from build123d import *

# Parameters (mm, degrees)
PAD066_DEPTH            = 57.4
POCKET083_DEPTH         = 4.5
SKETCH144_R             = 3.1
POCKET097_DEPTH         = 10
POCKET097_FACE16_W      = 10
POCKET097_FACE16_H      = 57.4
PAD073_DEPTH            = 6.35
SKETCH147_R             = 1.85
POCKET099_DEPTH         = 57.401
BODY017_PLACEMENT_ANGLE = 270


with BuildPart() as part:
    # Sketch126 → Pad066 (new body)
    with BuildSketch(Plane.XY):
        with BuildLine():
            Line((10, 10), (10, 60))
            Line((10, 60), (0, 60))
            Line((0, 60), (0, 0))
            add(Edge.make_bspline(
                [(0, 0), (45, -90), (90, 0)],
                knots=[0, 0, 0, 1, 1, 1], degree=2))
            Line((90, 0), (90, 60))
            Line((90, 60), (80, 60))
            Line((80, 60), (80, 10))
            add(Edge.make_bspline(
                [(10, 10), (45, -60), (80, 10)],
                knots=[0, 0, 0, 1, 1, 1], degree=2))
        make_face()
    extrude(amount=PAD066_DEPTH)

    # Sketch127 (on Face1 of Pad066) → Pocket083 (cut)
    with BuildSketch(Plane.YZ.offset(10)):
        Polygon((28.425, 33.679646), (25.55, 28.7), (28.425, 23.720354), (34.175, 23.720354), (37.05, 28.7), (34.175, 33.679646), align=None)
    extrude(amount=-POCKET083_DEPTH, mode=Mode.SUBTRACT)

    # Sketch144 (on Face13 of Pocket083) → Pocket097 (cut)
    with BuildSketch(Plane(origin=(0, 0, 0), x_dir=(0, -1, 0), z_dir=(-1, 0, 0))):
        with Locations((-31.3, 28.7)):
            Circle(SKETCH144_R)
    extrude(amount=-POCKET097_DEPTH, mode=Mode.SUBTRACT)

    # Pocket097 Face16 → Pad073 (add)
    with BuildSketch(Plane(origin=(85, 60, 28.7), x_dir=(1, 0, 0), z_dir=(0, 1, 0))):
        Rectangle(POCKET097_FACE16_W, POCKET097_FACE16_H)
    extrude(amount=PAD073_DEPTH)

    # Sketch147 (on Face16 of Pad073) → Pocket099 (cut, through all)
    with BuildSketch(Plane.XY.offset(57.4)):
        with Locations((85, 43.15)):
            Circle(SKETCH147_R)
        with Locations((85, 23.15)):
            Circle(SKETCH147_R)
    extrude(amount=-POCKET099_DEPTH, mode=Mode.SUBTRACT)


with BuildPart() as part_1:
    # Body017 placement: moved
    add(part.part.moved(Location((-71.28, -233.15, -123.29))).rotate(Axis((-71.28, -233.15, -123.29), (0, 1, 0)), BODY017_PLACEMENT_ANGLE))


solid = part_1.part
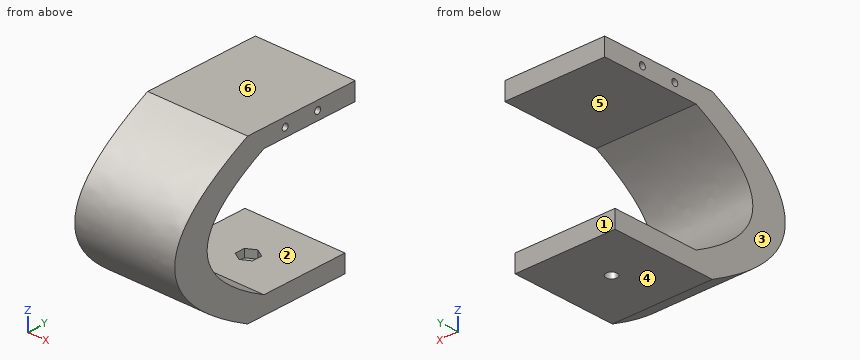
Verification items for the finished model (mm, model axes). Face numbers are marked on the shaded views. A direction names the side the tool comes from. Give positions to 0.01 mm unless a question says otherwise; leave off trailing zeros. Order: outer loops, then holes, each group sorted by start corner. A loop starts at its lowest first (then second) coordinate and runs counter-clockwise, first axis right, second up. Notation, with made-up numbers: M 81,12 L 114,12 A26 cw 114,34 Z; hole C 8,81.25 d9. An arc over 180 degrees is marked long. Answer as a JSON object with one key per item and string values. Group by question number.
1) Cross-section at C-C (x = -122.5). Give the number of separate pieces and of enclosed holes in the cut face, then the cut area to 3 significant figures.
2) Cross-section at A-A (y = -182). Enter the section's corners in (x, z), then the cut area to 3 significant figures.
3) Access from +Z, -Z, +X, -X, +Y, -Y to the whole of each face (thin tool, end or side, straight path). Record for the marked faces 1, 2 and 3.
4) Scan lines: line 1 along Z through (x, y) = (-99, -190); line 2 along Z through (x, y) = (-119, -195); line 3 along Y through (x, z) = (-84.5, -38.29). Record each from-to range of solid material in increasing order. Write a range as [from, to].
5) Cross-section at B-B (y = -201.85). Enter the section's corners in (x, z).
6) Depth check by flat-ended pin: pin 1 Ø3 at (x, z) = (-91, -88) entering from -Y; pin 2 Ø12 at (x, z) = (-88, -69) entering from -Y; pin 3 Ø4 at (x, z) = (-85, -97) entering from -Y (3 decimals). Enter the tip coordinate at first touch or a pass-through.
7) Mould release check, pull along Z, two halves, no side actions. Record for the marked faces 4, 5 and 6: released by +Z, released by -Z, zero draft, split by the parting line, or undercut.
Result sheet:
{
 "1": {"separate pieces": "1", "enclosed holes": "2", "area": "3,010 mm2"},
 "2": {"outline": "M -128.68,-123.29 L -71.28,-123.29 L -71.28,-113.29 L -128.68,-113.29 Z; M -128.68,-43.29 L -71.28,-43.29 L -71.28,-33.29 L -128.68,-33.29 Z", "area": "1,150 mm2"},
 "3": {"face 1": "-Z, +X, -X, +Y", "face 2": "+X, -X, +Y", "face 3": "+Z, -Z, -X, +Y, -Y"},
 "4": {"line 1": "z = [-123.29, -113.29], [-43.29, -40.14], [-36.44, -33.29]", "line 2": "z = [-123.29, -113.29], [-43.29, -33.29]", "line 3": "y = [-242.59, -211.85], [-208.15, -191.85], [-188.15, -166.8]"},
 "5": {"outline": "M -128.68,-123.29 L -103.08,-123.29 L -103.08,-117.79 L -104.96,-117.79 L -104.96,-113.29 L -128.68,-113.29 Z; M -128.68,-43.29 L -71.28,-43.29 L -71.28,-33.29 L -128.68,-33.29 Z; M -96.88,-123.29 L -71.28,-123.29 L -71.28,-113.29 L -95,-113.29 L -95,-117.79 L -96.88,-117.79 Z"},
 "6": {"pin 1": "stops at y = -276.65", "pin 2": "stops at y = -277.91", "pin 3": "stops at y = -271.945"},
 "7": {"face 4": "released by -Z", "face 5": "undercut", "face 6": "released by +Z"}
}
